Read the model definition and answer for the solid it produces. Units are mm, in the model's axes. A direction names the side the tool comes from. Give positions to 0.01 mm unless a question says otherwise; leave off trailing zeros. Order: outer loops, then holes, each group sorted by start corner. A loop starts at its lowest first (then second) coordinate and runs counter-clockwise, first axis right, second up. Notation, with made-up numbers: (-39, -27) -> (-28, -27) arc R34 cw to (-28, 4) -> close; hole circle Ø2 at (-13.5, 47.5). An arc over 180 degrees is marked (long way). Use one line per item in the form item = value.
```python
from build123d import *

# Parameters (mm, degrees)
F0_W     = 30
F0_H     = 40
F2_R     = 4
F3_DEPTH = 25
F4_DEPTH = 25


with BuildPart() as f1:
    # F0 (on Front) → F1 (revolve)
    with BuildSketch(Plane.XZ):
        Polygon((0, 105), (0, 70), (30, 70), (35, 70), (35, 105), align=None)
        with Locations((15, 50)):
            Rectangle(F0_W, F0_H)
        with BuildLine():
            Line((30, 30), (0, 30))
            Line((0, 30), (0, 0))
            ThreePointArc((0, 0), (21.2132034356, 8.7867965644), (30, 30))
        make_face()
    revolve(axis=Axis((0, 0, 50), (0, 0, -1)))

    # F2 (on Top) → F3 (join)
    with BuildSketch(Plane.XY):
        with BuildLine():
            ThreePointArc((14, 10), (10, 14), (6, 10))
            Line((6, 10), (10, 10))
            Line((10, 10), (10, 6))
            ThreePointArc((10, 6), (12.8284271247, 7.1715728753), (14, 10))
        make_face()
        with BuildLine():
            Line((-10, 10), (-6, 10))
            ThreePointArc((-6, 10), (-12.8284271247, 12.8284271247), (-10, 6))
            Line((-10, 6), (-10, 10))
        make_face()
        with BuildLine():
            ThreePointArc((14, -10), (12.8284271247, -7.1715728753), (10, -6))
            Line((10, -6), (10, -10))
            Line((10, -10), (6, -10))
            ThreePointArc((6, -10), (10, -14), (14, -10))
        make_face()
        with BuildLine():
            Line((-10, -10), (-10, -6))
            ThreePointArc((-10, -6), (-12.8284271247, -12.8284271247), (-6, -10))
            Line((-6, -10), (-10, -10))
        make_face()
        with BuildLine():
            Line((10, 10), (6, 10))
            ThreePointArc((6, 10), (7.1715728753, 7.1715728753), (10, 6))
            Line((10, 6), (10, 10))
        make_face()
        with BuildLine():
            ThreePointArc((-10, 6), (-7.1715728753, 7.1715728753), (-6, 10))
            Line((-6, 10), (-10, 10))
            Line((-10, 10), (-10, 6))
        make_face()
        with BuildLine():
            Line((10, -10), (10, -6))
            ThreePointArc((10, -6), (7.1715728753, -7.1715728753), (6, -10))
            Line((6, -10), (10, -10))
        make_face()
        with BuildLine():
            ThreePointArc((-6, -10), (-7.1715728753, -7.1715728753), (-10, -6))
            Line((-10, -6), (-10, -10))
            Line((-10, -10), (-6, -10))
        make_face()
        Circle(F2_R)
    extrude(amount=F3_DEPTH)

    # F4 (add): faces of the model
    f4_faces = [f1.faces().sort_by_distance(p)[0] for p in [
        (-10, -10, 0),
        (0, 0, 0),
        (-10, 10, 0),
        (10, -10, 0),
        (10, 10, 0),
    ]]
    extrude(f4_faces, amount=F4_DEPTH)


solid = f1.part
```
Item 1: Which of the six approach directions +Z, -Z, +X, -X, +Y, -Y give full straight-line access (tool end or side, diameter ignored) to faces 1 (the flat face through (-26, -16, 70)), 2 (the cylindrical face through (-28, 21, 88))?
Checks:
face_1 = -Z
face_2 = +Z, -Z
Item 2: The part is cut by section B-B on x = 17. Give the vertices of the cut face in (y, z), and give its area (3 significant figures).
Checks:
outline = (-30.59, 70) -> (-24.72, 70) -> (-24.72, 30) arc R24.72 ccw to (24.72, 30) -> (24.72, 70) -> (30.59, 70) -> (30.59, 105) -> (-30.59, 105) -> close
area = 5,080 mm²
Item 3: The part is cut by section D-D on y = -27. Give the vertices of the cut face in (x, z), and give its area (3 significant figures).
Checks:
outline = (-22.27, 70) -> (-13.08, 70) -> (-13.08, 30) arc R13.08 ccw to (13.08, 30) -> (13.08, 70) -> (22.27, 70) -> (22.27, 105) -> (-22.27, 105) -> close
area = 2,870 mm²
Item 4: Straight lines are drawn through the part: L1, parallel to Y at x = 10.5, z = -4.5; L2, parallel to Z at x = -30.5, y = -12; L3, parallel to Z at x = -2.5, y = 18. For each, find the intervals that lie inside material, in ascending order. Write a range as from..to.
Checks:
L1 = -13.97..-6.03, 6.03..13.97
L2 = 70..105
L3 = 6.13..105
Item 5: Given pin 1 Ø1.5 at (y, z) = (9.5, 46) entering from +X; pin 2 Ø4 at (x, z) = (18.5, 39) entering from +Y; pin 3 Ø10 at (y, z) = (14, -4.5) entering from -X, each flat-ended and moving along its own axis, determine where each tip first touches the part or whether it passes through.
Checks:
pin_1 = 28.7
pin_2 = 25.05
pin_3 = -14
Item 6: The part is cut by section A-A on y = -12. Give the vertices of the cut face in (x, z), and give its area (3 significant figures).
Checks:
outline = (-32.88, 70) -> (-27.5, 70) -> (-27.5, 30) arc R27.5 ccw to (-13.46, 6.03) -> (-13.46, -25) -> (-6.54, -25) -> (-6.54, 3.29) arc R27.5 ccw to (6.54, 3.29) -> (6.54, -25) -> (13.46, -25) -> (13.46, 6.03) arc R27.5 ccw to (27.5, 30) -> (27.5, 70) -> (32.88, 70) -> (32.88, 105) -> (-32.88, 105) -> close
area = 6,100 mm²
Item 7: The part is cut by section C-C on z = 45. Give the vertices of the cut face in (x, y), and give its area (3 significant figures).
Checks:
outline = circle Ø60 at (0, 0)
area = 2,830 mm²
